The drawing under review shows one solid part. Ordinate dimensions are in mm from its lowest x, y, z. Round coordinates to 2 decimals unless told otherwise and drop trailing zeros. Write each loop counter-clockwise with the first axis right and the second up, starting at its lowest first coordinate (ties: lowest second). Pieces come first, ordered by that corner, then holes.
Item 1: Add section A-A (x = 1.75). Give the boundary of the cut face in (y, z), plus the area to 3 significant figures.
Item 2: Clearance check with a flat-ended pin moving along its axis: pin 1 Ø3 at (x, z) = (3.925, 3.925) entering from +Y. State where the tip first meets the part, or that it passes through.
Item 3: Draft analysis for pull direction X (two halves, no side actions). For the marked faces 1 and 2, state which applies: +X half, -X half, draft (parallel to the pull), parting line (faces both ways), or undercut.
Item 4: To check wall thickness, follow L1, parallel to X at y = 3.45, z = 5.5; L2, parallel to Y at x = 5, z = 5.25; L3, parallel to Z at x = 2, y = 1.2. State the ranges of each line that lie inside material, in increasing order.
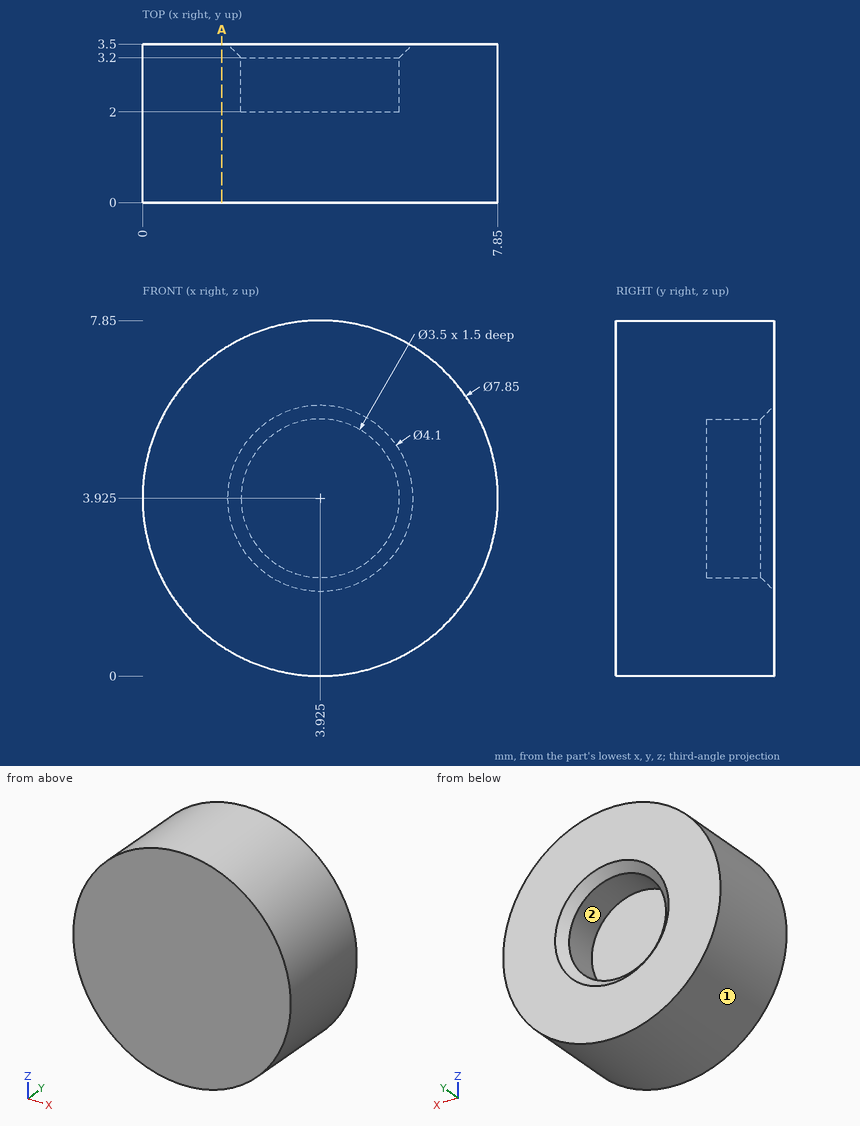
Numbers:
1. outline: (0, 0.66) - (3.5, 0.66) - (3.5, 7.19) - (0, 7.19) - close
1. area: 22.9 mm2
2. pin 1: stops at y = 2
3. face 1: parting line
3. face 2: undercut
4. L1: x = 0.33 to 2.69, 5.16 to 7.52
4. L2: y = 0 to 2
4. L3: z = 0.5 to 7.35
